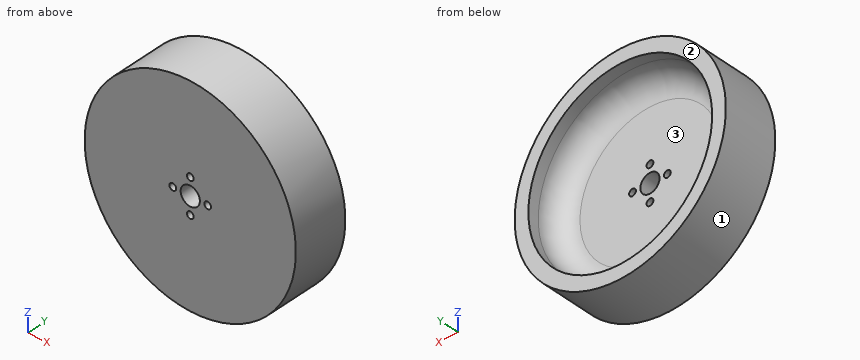
```python
from build123d import *

# Parameters (mm, degrees)
SKETCH001_R        = 1.236716
POCKET_DEPTH       = 241.432705
POLARPATTERN_COUNT = 4
FILLET_R           = 8


with BuildPart() as part:
    # Sketch → Revolution (revolve)
    with BuildSketch(Plane.YZ):
        Polygon((6.930658, 38.5), (26.930658, 38.5), (26.930658, 33.5), (14.930658, 33.5), (14.930658, 3.5), (6.930658, 3.5), align=None)
    revolve(axis=Axis((0, 0, 0), (0, 1, 0)))

    # Sketch001 (on Face6 of Revolution) → Pocket (cut, through all)
    with BuildSketch(Plane(origin=(0, 6.930658, 0), x_dir=(0, 0, -1), z_dir=(0, -1, 0))):
        with Locations((0, 6.35)):
            Circle(SKETCH001_R)
    pocket = extrude(amount=-POCKET_DEPTH, mode=Mode.SUBTRACT)

    # PolarPattern: Pocket ×4 about axis
    polarpattern_axis = Axis((0, 6.930658, 0), (0, -1, 0))
    for i in range(1, POLARPATTERN_COUNT):
        add(pocket.rotate(polarpattern_axis, i * 360 / POLARPATTERN_COUNT), mode=Mode.SUBTRACT)

    # Fillet
    fillet_edges = [part.edges().sort_by_distance(p)[0] for p in [
        (0, 14.930658, -33.5),
    ]]
    fillet(fillet_edges, radius=FILLET_R)


solid = part.part
```
Model file for the job. Use its own axes, mm. Face numbers are marked on the shaded views. Coordinates: 2 decimals unless noted, no trailing zeros. Write each loop counter-clockwise with the first axis right and the second up, starting at its lowest first coordinate (ties: lowest second). Pieces come first, ordered by that corner, then holes. Notation, with made-up numbers: (0.5, 88) - (45.5, 88) arc R6 cw to (45.5, 99) - close; hole circle Ø10 at (-22.75, 66.25). An arc over 180 degrees is marked (long way). Use a Markdown table: item, result. Add a question column.
Item 1: Drill centre lines: line 1 along X through (y, z) = (11.5, 0); line 2 along X through (y, z) = (20.75, 17); line 3 along Y through (x, z) = (18, -11). Where is each one in solid material? Low to high.
Item 2: Band-saw the part on C-C, the plane y = 19.75. Write the cut outline in (x, z).
Item 3: Band-saw the part on D-D, the plane y = 24.5. Write the cut outline in (x, z), and give its area (3 significant figures).
Item 4: Drop flat-ended pins along their axis: pin 1 (2 mm diameter, centred on x = 29.5, z = -9.5, fed in from +Y); pin 2 (4 mm diameter, centred on y = 20.5, z = 19, fed in from +X); pin 3 (1 mm diameter, centred on x = 17.5, z = -8.5, fed in from +Y); pin 4 (3 mm diameter, centred on x = 6.35, z = 0, fed in from -Y). Give the stop position or say it passes through.
Item 5: Band-saw the part on B-B, the plane y = 14. Write the cut outline in (x, z), and give its area (3 significant figures).
Item 6: Band-saw the part on A-A, the plane z = 0. Write the cut outline in (x, y).
Item 7: Two-plate mould, pull along X, no slides. Class the marked faces 1, 2 and 3: pulls with the +X half, pulls with the -X half, needs draft (parallel to the pull), parting line crosses it, or undercut.
A:
| question | item | result |
|---|---|---|
| 1 | line 1 | x = -38.5 to -7.59, -5.11 to -3.5, 3.5 to 5.11, 7.59 to 38.5 |
| 1 | line 2 | x = -34.54 to -28.51, 28.51 to 34.54 |
| 1 | line 3 | y = 6.93 to 14.93 |
| 2 | outline | circle Ø77 at (0, 0); hole circle Ø65.68 at (0, 0) |
| 3 | outline | circle Ø77 at (0, 0); hole circle Ø67 at (0, 0) |
| 3 | area | 1,130 mm² |
| 4 | pin 1 | stops at y = 18.26 |
| 4 | pin 2 | stops at x = 34.54 |
| 4 | pin 3 | stops at y = 14.93 |
| 4 | pin 4 | stops at y = 6.93 |
| 5 | outline | circle Ø77 at (0, 0); hole circle Ø2.47 at (-6.35, 0); hole circle Ø7 at (0, 0); hole circle Ø2.47 at (0, -6.35); hole circle Ø2.47 at (0, 6.35); hole circle Ø2.47 at (6.35, 0) |
| 5 | area | 4,600 mm² |
| 6 | outline | (-38.5, 6.93) - (-7.59, 6.93) - (-7.59, 14.93) - (-25.5, 14.93) arc R8 cw to (-33.5, 22.93) - (-33.5, 26.93) - (-38.5, 26.93) - close; (-5.11, 6.93) - (-3.5, 6.93) - (-3.5, 14.93) - (-5.11, 14.93) - close; (3.5, 6.93) - (5.11, 6.93) - (5.11, 14.93) - (3.5, 14.93) - close; (7.59, 6.93) - (38.5, 6.93) - (38.5, 26.93) - (33.5, 26.93) - (33.5, 22.93) arc R8 cw to (25.5, 14.93) - (7.59, 14.93) - close |
| 7 | face 1 | parting line crosses it |
| 7 | face 2 | needs draft |
| 7 | face 3 | undercut |
